For this review, take the finished solid that the model builds, in its own axes (mm). Face numbers are marked on the shaded views. A direction names the side the tool comes from. Round coordinates to 2 decimals unless told otherwise and drop trailing zeros. Order: outer loops, then holes, each group sorted by start corner. A loop starts at its lowest first (then second) coordinate and runs counter-clockwise, first axis right, second up. Notation, with made-up numbers: (73, -35) -> (95, -35) arc R18 cw to (95, -12) -> close; hole circle Ø2 at (53, -14). An arc over 180 degrees is marked (long way). Answer in a Markdown table with one row per item.
```python
from build123d import *

# Parameters (mm, degrees)
MODEL_R                 = 1.5
SALIENTE_EXTRUIR1_DEPTH = 3


with BuildPart() as part:
    # Model → Saliente-Extruir1 (new body)
    with BuildSketch(Plane.XY):
        with BuildLine():
            Line((149.34213351, 211.823953209), (158.34213351, 211.823953209))
            ThreePointArc((158.34213351, 211.823953209), (161.524114025, 210.505933724), (162.84213351, 207.323953209))
            Line((162.84213351, 207.323953209), (162.84213351, 198.323953209))
            ThreePointArc((162.84213351, 198.323953209), (158.34213351, 193.823953209), (153.84213351, 198.323953209))
            Line((153.84213351, 198.323953209), (153.84213351, 202.823953209))
            Line((153.84213351, 202.823953209), (149.34213351, 202.823953209))
            ThreePointArc((149.34213351, 202.823953209), (144.84213351, 207.323953209), (149.34213351, 211.823953209))
        make_face()
        with Locations((149.34213351, 207.323953209)):
            Circle(MODEL_R, mode=Mode.SUBTRACT)
        with Locations((158.34213351, 207.323953209)):
            Circle(MODEL_R, mode=Mode.SUBTRACT)
        with Locations((158.34213351, 198.323953209)):
            Circle(MODEL_R, mode=Mode.SUBTRACT)
    extrude(amount=SALIENTE_EXTRUIR1_DEPTH)


solid = part.part
```
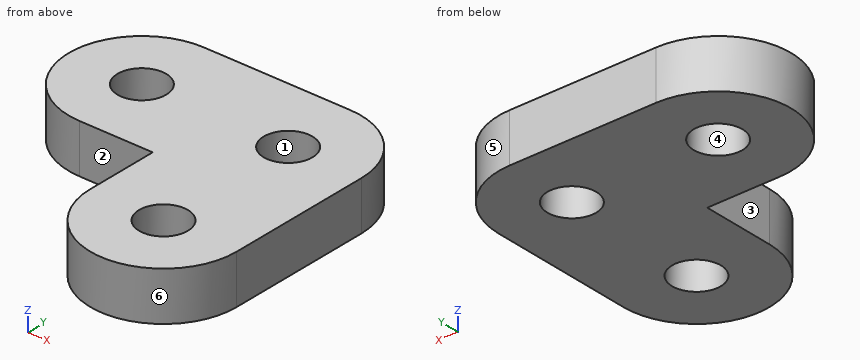
Q1. The part is to be moulded in two halves that separate along X. For the marked faces 3, 4, 5 and 6, say which applies: +X half, -X half, draft (parallel to the pull), parting line (faces both ways), or undercut.
Answer key:
| item | result |
|---|---|
| face 3 | -X half |
| face 4 | undercut |
| face 5 | +X half |
| face 6 | parting line |
Q2. To check wall thickness, follow probe 1 along X at (y, z) = (207.75, 2.4); probe 2 along X at (y, z) = (202, 0.2); probe 3 along X at (y, z) = (199.25, 0.85). State the ranges of each line that lie inside material, in increasing order.
Answer key:
| item | result |
|---|---|
| probe 1 | x = 144.86 to 147.9, 150.78 to 156.9, 159.78 to 162.82 |
| probe 2 | x = 153.84 to 162.84 |
| probe 3 | x = 153.84 to 157.16, 159.52 to 162.84 |
Q3. Take a section at C-C, the plane x = 159.5. Write out the cut boundary in (y, z).
Answer key:
| item | result |
|---|---|
| outline | (193.98, 0) -> (197.37, 0) -> (197.37, 3) -> (193.98, 3) -> close; (199.28, 0) -> (206.37, 0) -> (206.37, 3) -> (199.28, 3) -> close; (208.28, 0) -> (211.67, 0) -> (211.67, 3) -> (208.28, 3) -> close |
Q4. Tool access review of the marked faces 1 and 2: name each direction out of +Z, -Z, +X, -X, +Y, -Y from which nothing blocks a thin tool from reaching the whole face with its end or side.
Answer key:
| item | result |
|---|---|
| face 1 | +Z, -Z |
| face 2 | +Z, -Z, -X, -Y |
Q5. Clearance check with flat-ended pins moving along their axes: pin 1 Ø6 at (x, y) = (147, 200.5) entering from +Z; pin 2 Ø1.5 at (y, z) = (199.5, 2) entering from -X. State where each tip first meets the part, or that it passes through.
Answer key:
| item | result |
|---|---|
| pin 1 | stops at z = 3 |
| pin 2 | stops at x = 153.84 |
Q6. Take a section at B-B, the plane y = 208.25. Write out the cut boundary in (x, z).
Answer key:
| item | result |
|---|---|
| outline | (144.94, 0) -> (148.16, 0) -> (148.16, 3) -> (144.94, 3) -> close; (150.52, 0) -> (157.16, 0) -> (157.16, 3) -> (150.52, 3) -> close; (159.52, 0) -> (162.75, 0) -> (162.75, 3) -> (159.52, 3) -> close |
Q7. Take a section at D-D, the plane y = 210.5. Write out the cut boundary in (x, z).
Answer key:
| item | result |
|---|---|
| outline | (146.15, 0) -> (161.53, 0) -> (161.53, 3) -> (146.15, 3) -> close |
Q8. Take a section at A-A, the plane z = 0.55. Write out the cut boundary in (x, y).
Answer key:
| item | result |
|---|---|
| outline | (149.34, 202.82) -> (153.84, 202.82) -> (153.84, 198.32) arc R4.5 ccw to (162.84, 198.32) -> (162.84, 207.32) arc R4.5 ccw to (158.34, 211.82) -> (149.34, 211.82) arc R4.5 ccw to start; hole circle Ø3 at (149.34, 207.32); hole circle Ø3 at (158.34, 198.32); hole circle Ø3 at (158.34, 207.32) |
